The listing builds one solid part. Answer for the finished solid, in the listing's coordinates (mm). A direction names the side the tool comes from. Coordinates: 2 decimals unless noted, no trailing zeros. Loops run counter-clockwise (first coordinate to the right, second up) from the corner with the lowest first, then second, coordinate; pieces in that order, holes last. Notation, with made-up numbers: M 64.25,-29 L 98.25,-29 A21 cw 98.25,-4 Z; hole C 15.25,-30.75 d11. An arc over 180 degrees is marked long. Answer as a JSON object with one key per item and string values. Group by question number.
1. Determine the mould class of faces 4 (the face through (-34, -16, 50.719)), 5 (the face through (49.684, -26.048, 49.198)), 6 (the face through (-40, -27, -54)), 7 (the face through (-18.316, -26.048, 49.198)) for opening direction Y: released by +Y, released by -Y, zero draft, split by the parting line, or undercut.
2. A cutting plane is placed at B-B on z = -46.5. Give the vertices of the cut face in (x, y).
3. Straight lines are drawn through the part: L1, parallel to Y at x = -49.25, z = 50; L2, parallel to Z at x = 27, y = -26.5; L3, parallel to Y at x = 18, z = 49. For each, find the intervals that lie inside material, in ascending order.
4. A cutting plane is placed at C-C on x = -49.25. Give the vertices of the cut face in (y, z).
5. A cutting plane is placed at D-D on y = -5. State how many separate pieces and enclosed holes the cut face has, and give its area (3 significant figures).
6. For faces 1 (the face through (-49.684, -29.952, 49.198)), 2 (the face through (25, 0.2, -38.7)), 3 (the face through (0, 1, 47.719)), determine the directions among +Z, -Z, +X, -X, +Y, -Y from which every point of the face is accessible in a straight line to the end or side of a thin tool.
7. A cutting plane is placed at A-A on y = -22. Give the vertices of the cut face in (x, z).
8. Given pin 1 (3 mm diameter, centred on x = -15, y = -9, fed in from -Z); pin 2 (6 mm diameter, centred on x = -20, z = -1.5, fed in from -Y); pin 3 (2.5 mm diameter, centred on x = 39.5, z = -54, fed in from -Y), each flat-ended and moving along its own axis, determine where each tip first touches the part or whether it passes through.
from build123d import *

# Parameters (mm, degrees)
BOSS_EXTRUDE1_DEPTH = 3
SKETCH4_W           = 42
SKETCH4_H           = 39
SKETCH4_R           = 2
BOSS_EXTRUDE2_DEPTH = 3
SKETCH5_W           = 30
SKETCH5_H           = 30
SKETCH5_R           = 2
BOSS_EXTRUDE3_DEPTH = 3


with BuildPart() as part:
    # Sketch2 → Boss-Extrude1 (new body)
    with BuildSketch(Plane(origin=(0, 0, 0), x_dir=(1, 0, 0), z_dir=(0, 1, 0))):
        Polygon((-55, 52.280903811), (-55, -47.719096189), (55, -47.719096189), (55, 52.280903811), (25, 52.280903811), (25, 2.280903811), (-25, 2.280903811), (-25, 52.280903811), align=None)
    extrude(amount=BOSS_EXTRUDE1_DEPTH)

    # Sketch4 → Boss-Extrude2 (add)
    # profile 1 of 2: a face of its own
    with BuildSketch(Plane.XY.offset(47.719096189)):
        with Locations((-34, -16.5)):
            Rectangle(SKETCH4_W, SKETCH4_H)
        with Locations((-18.75, -5)):
            Circle(SKETCH4_R, mode=Mode.SUBTRACT)
        with Locations(Location((-49.25, -5, 0), (0, 0, 180))):
            Circle(SKETCH4_R, mode=Mode.SUBTRACT)
        with Locations(Location((-18.75, -28, 0), (0, 0, 180))):
            Circle(SKETCH4_R, mode=Mode.SUBTRACT)
        with Locations((-49.25, -28)):
            Circle(SKETCH4_R, mode=Mode.SUBTRACT)
    # profile 2 of 2: a face of its own
    with BuildSketch(Plane.XY.offset(47.719096189)):
        with Locations((34, -16.5)):
            Rectangle(SKETCH4_W, SKETCH4_H)
        with Locations((49.25, -5)):
            Circle(SKETCH4_R, mode=Mode.SUBTRACT)
        with Locations(Location((49.25, -28, 0), (0, 0, 180))):
            Circle(SKETCH4_R, mode=Mode.SUBTRACT)
        with Locations(Location((18.75, -5, 0), (0, 0, 180))):
            Circle(SKETCH4_R, mode=Mode.SUBTRACT)
        with Locations((18.75, -28)):
            Circle(SKETCH4_R, mode=Mode.SUBTRACT)
    extrude(amount=BOSS_EXTRUDE2_DEPTH)

    # Sketch5 → Boss-Extrude3 (add)
    # profile 1 of 2: a face of its own
    with BuildSketch(Plane(origin=(0, 0, -52.280903811), x_dir=(-1, 0, 0), z_dir=(0, 0, -1))):
        with Locations((40, -12)):
            Rectangle(SKETCH5_W, SKETCH5_H)
        with Locations((40, -12)):
            Circle(SKETCH5_R, mode=Mode.SUBTRACT)
    # profile 2 of 2: a face of its own
    with BuildSketch(Plane(origin=(0, 0, -52.280903811), x_dir=(-1, 0, 0), z_dir=(0, 0, -1))):
        with Locations((-40, -12)):
            Rectangle(SKETCH5_W, SKETCH5_H)
        with Locations(Location((-40, -12, 0), (0, 0, 180))):
            Circle(SKETCH5_R, mode=Mode.SUBTRACT)
    extrude(amount=BOSS_EXTRUDE3_DEPTH)


solid = part.part
From the geometry:
{
 "1": {"face 4": "zero draft", "face 5": "undercut", "face 6": "released by -Y", "face 7": "undercut"},
 "2": {"outline": "M -55,0 L -25,0 L -25,3 L -55,3 Z; M 25,0 L 55,0 L 55,3 L 25,3 Z"},
 "3": {"L1": "y = -36 to -30, -26 to -7, -3 to 3", "L2": "z = -55.28 to -52.28, 47.72 to 50.72", "L3": "y = -36 to -29.85, -26.15 to -6.85, -3.15 to 3"},
 "4": {"outline": "M -36,47.72 L -30,47.72 L -30,50.72 L -36,50.72 Z; M -27,-55.28 L 3,-55.28 L 3,50.72 L -3,50.72 L -3,47.72 L 0,47.72 L 0,-52.28 L -27,-52.28 Z; M -26,47.72 L -7,47.72 L -7,50.72 L -26,50.72 Z"},
 "5": {"separate pieces": "8", "enclosed holes": "0", "area": "384 mm²"},
 "6": {"face 1": "+Z", "face 2": "-Z, +Y, -Y", "face 3": "+Z, +Y, -Y"},
 "7": {"outline": "M -55,-55.28 L -25,-55.28 L -25,-52.28 L -55,-52.28 Z; M -55,47.72 L -13,47.72 L -13,50.72 L -55,50.72 Z; M 13,47.72 L 55,47.72 L 55,50.72 L 13,50.72 Z; M 25,-55.28 L 55,-55.28 L 55,-52.28 L 25,-52.28 Z"},
 "8": {"pin 1": "stops at z = 47.72", "pin 2": "stops at y = 0", "pin 3": "stops at y = -27"}
}
